from build123d import *

# Parameters (mm, degrees)
SKETCH1_R           = 15
BOSS_EXTRUDE1_DEPTH = 115
BOSS_EXTRUDE2_DEPTH = 5
SKETCH3_R           = 13.25
SKETCH3_R_2         = 13
CUT_EXTRUDE1_DEPTH  = 0.5
SKETCH4_R           = 10
CUT_EXTRUDE2_DEPTH  = 125.128965193
SKETCH5_R           = 1.5
BOSS_EXTRUDE3_DEPTH = 10.35


with BuildPart() as part:
    # Sketch1 → Boss-Extrude1 (new body)
    with BuildSketch(Plane(origin=(0, 0, 0), x_dir=(1, 0, 0), z_dir=(0, 1, 0))):
        with Locations(Location((0, 0, 0), (0, 0, 270))):
            Circle(SKETCH1_R)
    extrude(amount=BOSS_EXTRUDE1_DEPTH)

    # Sketch2 → Boss-Extrude2 (add)
    with BuildSketch(Plane(origin=(0, 115, 0), x_dir=(1, 0, 0), z_dir=(0, 1, 0))):
        with BuildLine():
            Line((-1.5, 20.5), (1.5, 20.5))
            Line((1.5, 20.5), (1.5, 22.449944321))
            ThreePointArc((1.5, 22.449944321), (15.909902577, 15.909902577), (22.449944321, 1.5))
            Line((22.449944321, 1.5), (20.5, 1.5))
            Line((20.5, 1.5), (20.5, -1.5))
            Line((20.5, -1.5), (22.449944321, -1.5))
            ThreePointArc((22.449944321, -1.5), (15.909902577, -15.909902577), (1.5, -22.449944321))
            Line((1.5, -22.449944321), (1.5, -20.5))
            Line((1.5, -20.5), (-1.5, -20.5))
            Line((-1.5, -20.5), (-1.5, -22.449944321))
            ThreePointArc((-1.5, -22.449944321), (-15.909902577, -15.909902577), (-22.449944321, -1.5))
            Line((-22.449944321, -1.5), (-20.5, -1.5))
            Line((-20.5, -1.5), (-20.5, 1.5))
            Line((-20.5, 1.5), (-22.449944321, 1.5))
            ThreePointArc((-22.449944321, 1.5), (-15.909902577, 15.909902577), (-1.5, 22.449944321))
            Line((-1.5, 22.449944321), (-1.5, 20.5))
        make_face()
    extrude(amount=BOSS_EXTRUDE2_DEPTH)

    # Sketch3 → Cut-Extrude1 (cut)
    with BuildSketch(Plane(origin=(0, 120, 0), x_dir=(1, 0, 0), z_dir=(0, 1, 0))):
        with Locations(Location((0, 0, 0), (0, 0, 270))):
            Circle(SKETCH3_R)
        with Locations(Location((0, 0, 0), (0, 0, 270))):
            Circle(SKETCH3_R_2, mode=Mode.SUBTRACT)
    extrude(amount=-CUT_EXTRUDE1_DEPTH, mode=Mode.SUBTRACT)

    # Sketch4 → Cut-Extrude2 (cut, through all)
    with BuildSketch(Plane(origin=(0, 120, 0), x_dir=(1, 0, 0), z_dir=(0, 1, 0))):
        with Locations(Location((0, 0, 0), (0, 0, 270))):
            Circle(SKETCH4_R)
    extrude(amount=-CUT_EXTRUDE2_DEPTH, mode=Mode.SUBTRACT)

    # Sketch5 → Boss-Extrude3 (add, symmetric)
    with BuildSketch(Plane(origin=(0, 0, 0), x_dir=(0, 0, -1), z_dir=(1, 0, 0))):
        with Locations(Location((0, 97.584149944, 0), (0, 0, 180))):
            Circle(SKETCH5_R)
    extrude(amount=BOSS_EXTRUDE3_DEPTH, both=True)


solid = part.part
CAD build for the part. Positions are in the model's coordinates, mm. A direction names the side the tool comes from. Give positions to 0.01 mm unless a question says otherwise; leave off trailing zeros. Loops run counter-clockwise (first coordinate to the right, second up) from the corner with the lowest first, then second, coordinate; pieces in that order, holes last. Notation, with made-up numbers: M 11,64 L 59,64 A22 ccw 59,92 Z; hole C 73.5,74.5 d1. An arc over 180 degrees is marked long. Answer in a Markdown table with one row per item. Add a question column.
Item 1: Band-saw the part on C-C on z = -7.5. Give the cut face in (x, y), then the cut area to 3 significant figures.
Item 2: Drop flat-ended pins along their axis: P1, Ø1.5, axis at y = 116.5, z = -0.5, coming from the -X side; P2, Ø2, axis at x = -1.5, y = 44.5, coming from the -Z side; P3, Ø3, axis at x = 6, y = 82.5, coming from the -Z side. Give the stop position or say it passes through.
Item 3: Tool access for faces 5 (the face through (0, 117, -20.5)), 6 (the face through (13.137, 119.754, -1.725)), 7 (the face through (-20.5, 117, 0)), 8 (the face through (0.14, 96.32, 0.81)), 9 (the face through (0.66, 56.695, -14.985)): list every direction of +Z, -Z, +X, -X, +Y, -Y with a clear straight run to the whole face (end or side of a thin tool).
Item 4: Band-saw the part on D-D on y = 32. Give the cut face in (x, z).
Item 5: Mould opens along Z. For faces 1 (the face through (-9.76, 60.84, -2.17)), 2 (the face through (20.5, 117, 0)), 3 (the face through (15.75, 117.46, -16.07)), 4 (the face through (-5, 115, 15)) say: +Z half, -Z half, draft (parallel to the pull), parting line (faces both ways), or undercut.
Item 6: Band-saw the part on B-B on x = 0. Give the cut face in (y, z).
Item 7: Band-saw the part on A-A on z = 0. Give the cut face in (x, y).
Item 8: Probe probe 1 along Y at (x, z) = (-12, 13); probe 2 along Z at (x, y) = (9, 62.5); probe 3 along Z at (x, y) = (-2.5, 15). List the from-to ranges inside material, lowest first.
Reply:
| question | item | result |
|---|---|---|
| 1 | outline | M -21.21,115 L -12.99,115 L -12.99,0 L -6.61,0 L -6.61,120 L -10.62,120 L -10.62,119.5 L -10.92,119.5 L -10.92,120 L -21.21,120 Z; M 6.61,0 L 12.99,0 L 12.99,115 L 21.21,115 L 21.21,120 L 10.92,120 L 10.92,119.5 L 10.62,119.5 L 10.62,120 L 6.61,120 Z |
| 1 | area | 1,610 mm^2 |
| 2 | P1 | stops at x = -20.5 |
| 2 | P2 | stops at z = -14.99 |
| 2 | P3 | stops at z = -14.31 |
| 3 | face 5 | -Z, +Y, -Y |
| 3 | face 6 | +Y |
| 3 | face 7 | -X, +Y, -Y |
| 3 | face 8 | none |
| 3 | face 9 | -Y |
| 4 | outline | C 0,0 d30; hole C 0,0 d20 |
| 5 | face 1 | undercut |
| 5 | face 2 | undercut |
| 5 | face 3 | -Z half |
| 5 | face 4 | draft |
| 6 | outline | M 0,-15 L 115,-15 L 115,-20.5 L 120,-20.5 L 120,-13.25 L 119.5,-13.25 L 119.5,-13 L 120,-13 L 120,-10 L 0,-10 Z; M 0,10 L 120,10 L 120,13 L 119.5,13 L 119.5,13.25 L 120,13.25 L 120,20.5 L 115,20.5 L 115,15 L 0,15 Z; C 97.58,0 d3 |
| 7 | outline | M -20.5,115 L -15,115 L -15,0 L -10,0 L -10,96.08 L 10,96.08 L 10,0 L 15,0 L 15,115 L 20.5,115 L 20.5,120 L 13.25,120 L 13.25,119.5 L 13,119.5 L 13,120 L 10,120 L 10,99.08 L -10,99.08 L -10,120 L -13,120 L -13,119.5 L -13.25,119.5 L -13.25,120 L -20.5,120 Z |
| 8 | probe 1 | y = 115 to 120 |
| 8 | probe 2 | z = -12 to -4.36, 4.36 to 12 |
| 8 | probe 3 | z = -14.79 to -9.68, 9.68 to 14.79 |
